from build123d import *

# Parameters (mm, degrees)
SKETCH1_R           = 27.5
BOSS_EXTRUDE1_DEPTH = 100
BOSS_EXTRUDE3_START = -7
SKETCH6_R           = 16
BOSS_EXTRUDE3_DEPTH = 12


with BuildPart() as part:
    # Sketch1 → Boss-Extrude1 (new body)
    with BuildSketch(Plane(origin=(0, 0, 0), x_dir=(1, 0, 0), z_dir=(0, 1, 0))):
        Circle(SKETCH1_R)
    extrude(amount=BOSS_EXTRUDE1_DEPTH)

    # Sketch6 → Boss-Extrude3 (add)
    with BuildSketch(Plane.XY.offset(10.010953).offset(BOSS_EXTRUDE3_START)):
        with BuildLine():
            Line((22.5, 0), (-22.5, 0))
            Line((-22.5, 0), (-22.5, -30))
            ThreePointArc((-22.5, -30), (0, -52.508858033), (22.5, -30))
            Line((22.5, -30), (22.5, 0))
        make_face()
        with Locations((0, -30.00885629)):
            Circle(SKETCH6_R, mode=Mode.SUBTRACT)
    boss_extrude3 = extrude(amount=BOSS_EXTRUDE3_DEPTH)

    # Mirror1: Boss-Extrude3 across plane
    add(boss_extrude3.mirror(Plane.XY))


solid = part.part
Work out the finished part from the listing and answer in its coordinate system (mm). A direction names the side the tool comes from. Coordinates: 2 decimals unless noted, no trailing zeros. Write each loop counter-clockwise with the first axis right and the second up, starting at its lowest first coordinate (ties: lowest second). Pieces come first, ordered by that corner, then holes. Notation, with made-up numbers: M 56,73.25 L 95,73.25 A15 ccw 95,95.25 Z; hole C 30.5,46 d10. An arc over 180 degrees is marked long. Use one line per item in the form item = value. Start each with the question number.
1. Straight lines are drawn through the part: probe 1 along Z at (x, y) = (-0.5, -8); probe 2 along Y at (x, z) = (0, -6.5); probe 3 along Y at (x, z) = (-13.5, 4). For each, find the intervals that lie inside material, in ascending order. Write a range as from..to.
2. The part is cut by section A-A (x = 0). Give the vertices of the cut face in (y, z).
3. Each of these flat-tipped pins is pushed along its axis until it touches: P1, Ø3, axis at x = 16, z = -2.5, coming from the -Y side; P2, Ø9.5, axis at y = -19, z = -9.5, coming from the +X side; P3, Ø3.5, axis at y = -15.5, z = 12, coming from the -X side; P4, Ø13.5, axis at x = 2, y = -38.5, coming from the -Z side. Where does it stop, or does it pass through?
4. The mould has two halves that part along Z. Classify faces 5 (the face through (-5.961, 49.3, 26.846)), 6 (the face through (-5, -14, -3.011)), 7 (the face through (0, 100, 0)): released by +Z, released by -Z, zero draft, split by the parting line, or undercut.
5. The part is cut by section B-B (z = 9). Give the vertices of the cut face in (x, y), plus the area to 3 significant figures.
6. The part is cut by section D-D (z = 0). Give the vertices of the cut face in (x, y).
7. A tool of negligible diameter and unlimited length cuts with its end or side. For faces 1 (the face through (-5, -14, -15.011)), 2 (the face through (-5, -14, 15.011)), 3 (the face through (22.5, -15, 9)), 4 (the face through (-22.5, -15, 9)), from which of +Z, -Z, +X, -X, +Y, -Y can it reach the whole face along a straight path? Write none if from no direction.
8. The part is cut by section C-C (y = -18.5). Give the vertices of the cut face in (x, z).
Evaluation:
q1.probe_1 = -15.01..-3.01, 3.01..15.01
q1.probe_2 = -52.51..-46.01, -14.01..100
q1.probe_3 = -48.01..-38.6, -21.42..100
q2.outline = M -52.51,-15.01 L -46.01,-15.01 L -46.01,-3.01 L -52.51,-3.01 Z; M -52.51,3.01 L -46.01,3.01 L -46.01,15.01 L -52.51,15.01 Z; M -14.01,-15.01 L 0,-15.01 L 0,-27.5 L 100,-27.5 L 100,27.5 L 0,27.5 L 0,15.01 L -14.01,15.01 L -14.01,3.01 L 0,3.01 L 0,-3.01 L -14.01,-3.01 Z
q3.P1 = -47.14
q3.P2 = 22.5
q3.P3 = -22.5
q3.P4 = through
q4.face_5 = split by the parting line
q4.face_6 = undercut
q4.face_7 = zero draft
q5.outline = M -25.99,0 L -22.5,0 L -22.5,-30 A22.5 ccw 22.5,-30 L 22.5,0 L 25.99,0 L 25.99,100 L -25.99,100 Z; hole C 0,-30.01 d32
q5.area = 6,540 mm^2
q6.outline = M -27.5,0 L 27.5,0 L 27.5,100 L -27.5,100 Z
q7.face_1 = -Z, +X, -X, -Y
q7.face_2 = +Z, +X, -X, -Y
q7.face_3 = +Z, -Z, +X, -Y
q7.face_4 = +Z, -Z, -X, -Y
q8.outline = M -22.5,-15.01 L -11.12,-15.01 L -11.12,-3.01 L -22.5,-3.01 Z; M -22.5,3.01 L -11.12,3.01 L -11.12,15.01 L -22.5,15.01 Z; M 11.12,-15.01 L 22.5,-15.01 L 22.5,-3.01 L 11.12,-3.01 Z; M 11.12,3.01 L 22.5,3.01 L 22.5,15.01 L 11.12,15.01 Z
